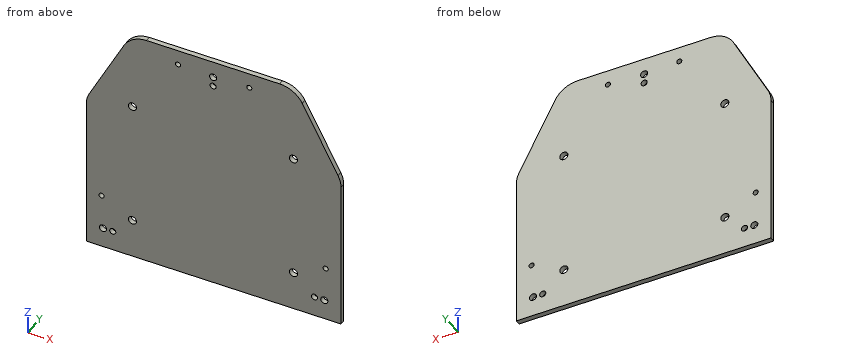
```python
from build123d import *

# Parameters (mm, degrees)
RESSALTO_EXTRUS_O4_DEPTH = 5
ESBO_O2_R                = 2.5
CORTE_EXTRUS_O1_DEPTH    = 5
ESBO_O3_R                = 4
CORTE_EXTRUS_O2_DEPTH    = 5
ESBO_O4_R                = 3.5
ESBO_O4_R_2              = 3
CORTE_EXTRUS_O3_DEPTH    = 10


with BuildPart() as part:
    # Esboço1 → Ressalto-extrusão4 (new body)
    with BuildSketch(Plane(origin=(0, 0, 0), x_dir=(1, 0, 0), z_dir=(0, 1, 0))):
        with BuildLine():
            Line((649.267355398, 124.203004206), (399.267355398, 124.203004206))
            Line((399.267355398, 124.203004206), (399.267355398, 84.203004206))
            Line((399.267355398, 84.203004206), (399.267355398, -25.823867232))
            ThreePointArc((399.267355398, -25.823867232), (399.994184105, -31.80827659), (402.132407827, -37.444714707))
            Line((402.132407827, -37.444714707), (436.243300323, -102.417843269))
            ThreePointArc((436.243300323, -102.417843269), (445.44614031, -112.192336255), (458.378247894, -115.796995794))
            Line((458.378247894, -115.796995794), (504.267355398, -115.796995794))
            Line((504.267355398, -115.796995794), (544.267355398, -115.796995794))
            Line((544.267355398, -115.796995794), (589.136322684, -115.796995794))
            ThreePointArc((589.136322684, -115.796995794), (602.010224955, -112.227409704), (611.207767027, -102.53800702))
            Line((611.207767027, -102.53800702), (646.338799741, -36.496622823))
            ThreePointArc((646.338799741, -36.496622823), (648.524169993, -30.805979), (649.267355398, -24.755611597))
            Line((649.267355398, -24.755611597), (649.267355398, 84.203004206))
            Line((649.267355398, 84.203004206), (649.267355398, 124.203004206))
        make_face()
    extrude(amount=RESSALTO_EXTRUS_O4_DEPTH)

    # Esboço2 → Corte-extrusão1 (cut)
    with BuildSketch(Plane(origin=(0, 5, 0), x_dir=(1, 0, 0), z_dir=(0, 1, 0))):
        with Locations(Location((559.267355398, -100.796995794, 0), (0, 0, 270))):
            Circle(ESBO_O2_R)
        with Locations(Location((489.267355398, -100.796995794, 0), (0, 0, 270))):
            Circle(ESBO_O2_R)
        with Locations(Location((634.267355398, 69.203004206, 0), (0, 0, 270))):
            Circle(ESBO_O2_R)
        with Locations(Location((414.267355398, 69.203004206, 0), (0, 0, 270))):
            Circle(ESBO_O2_R)
    extrude(amount=-CORTE_EXTRUS_O1_DEPTH, mode=Mode.SUBTRACT)

    # Esboço3 → Corte-extrusão2 (cut)
    with BuildSketch(Plane(origin=(0, 5, 0), x_dir=(1, 0, 0), z_dir=(0, 1, 0))):
        with Locations(Location((602.59531099, 85.223299861, 0), (0, 0, 270))):
            Circle(ESBO_O3_R)
        with Locations(Location((444.59531099, 85.223299861, 0), (0, 0, 270))):
            Circle(ESBO_O3_R)
        with Locations(Location((602.59531099, -38.776700139, 0), (0, 0, 270))):
            Circle(ESBO_O3_R)
        with Locations(Location((444.59531099, -38.776700139, 0), (0, 0, 270))):
            Circle(ESBO_O3_R)
    extrude(amount=-CORTE_EXTRUS_O2_DEPTH, mode=Mode.SUBTRACT)

    # Esboço4 → Corte-extrusão3 (cut)
    with BuildSketch(Plane(origin=(0, 5, 0), x_dir=(1, 0, 0), z_dir=(0, 1, 0))):
        with Locations(Location((523.757285289, -99.396995794, 0), (0, 0, 270))):
            Circle(ESBO_O4_R)
        with Locations(Location((632.867355398, 104.203004206, 0), (0, 0, 270))):
            Circle(ESBO_O4_R)
        with Locations(Location((415.667355398, 104.203004206, 0), (0, 0, 270))):
            Circle(ESBO_O4_R)
        with Locations(Location((623.267355398, 104.203004206, 0), (0, 0, 270))):
            Circle(ESBO_O4_R_2)
        with Locations(Location((425.267355398, 104.203004206, 0), (0, 0, 270))):
            Circle(ESBO_O4_R_2)
        with Locations(Location((523.757285289, -89.796995794, 0), (0, 0, 270))):
            Circle(ESBO_O4_R_2)
    extrude(amount=-CORTE_EXTRUS_O3_DEPTH, mode=Mode.SUBTRACT)


solid = part.part
```
CAD build for the part. Positions are in the model's coordinates, mm. Coordinates: 2 decimals unless noted, no trailing zeros. Write each loop counter-clockwise with the first axis right and the second up, starting at its lowest first coordinate (ties: lowest second). Pieces come first, ordered by that corner, then holes. Notation, with made-up numbers: (10.5, 12.5) -> (30.5, 12.5) arc R14 ccw to (30.5, 34.5) -> close; hole circle Ø7 at (43, 14.5). An arc over 180 degrees is marked (long way). Return JSON: item names as keys, results as strings. Group by question number.
Q1. Cut at B-B, the plane z = 77.5. Give the cut face in (x, y).
Q2. Flat gauge pin, fed straight in: pin 1 (1 mm diameter, centred on x = 521, z = -44, fed in from -Y). Where does the tip first touch, or does it go through?
Q3. Cut at A-A, the plane y = 2.65. State how many separate pieces and enclosed holes the cut face has, then the cut area to 3 significant figures.
Q4. Drill centre lines: line 1 (X direction, y = 3.55, z = -69.5); line 2 (Z direction, x = 445, y = 0.5); line 3 (X direction, y = 1.65, z = -106.5). Where is each one in solid material? Low to high.
Returned:
{
 "1": {"outline": "(423.16, 0) -> (624.53, 0) -> (624.53, 5) -> (423.16, 5) -> close"},
 "2": {"pin 1": "stops at y = 0"},
 "3": {"separate pieces": "1", "enclosed holes": "14", "area": "55,700 mm2"},
 "4": {"line 1": "x = 399.27 to 411.79, 416.75 to 631.79, 636.75 to 649.27", "line 2": "z = -124.2 to -89.2, -81.24 to 34.8, 42.76 to 111.92", "line 3": "x = 399.27 to 413.03, 418.31 to 423.34, 427.2 to 621.34, 625.2 to 630.23, 635.51 to 649.27"}
}
